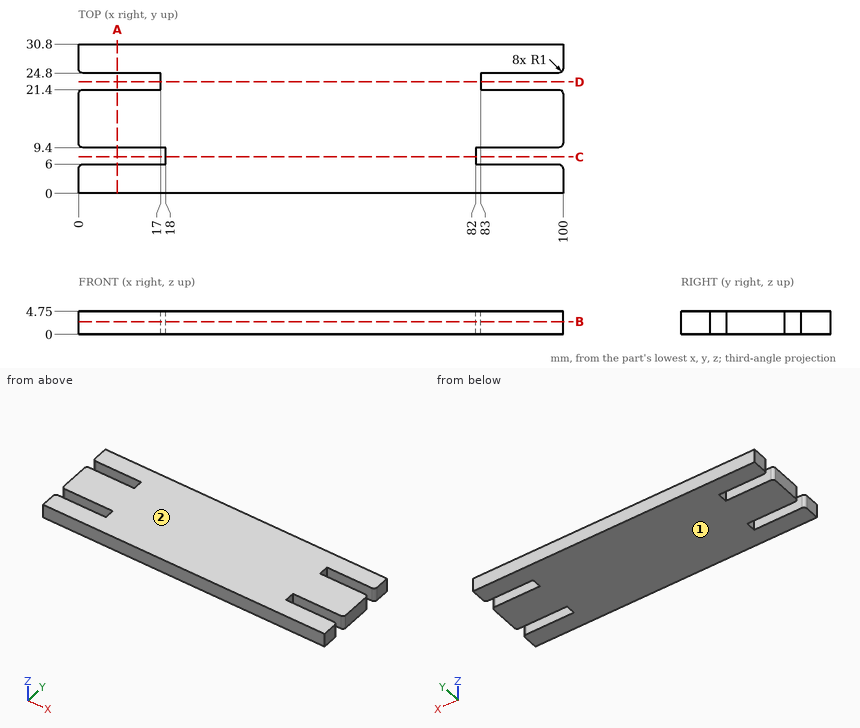
Verification items for this drawing (mm, ordinates from the low corner). Coordinates: 2 decimals unless noted, no trailing zeros. Write each loop counter-clockwise with the first axis right and the second up, starting at its lowest first coordinate (ties: lowest second). Pieces come first, ordered by that corner, then holes. Notation, with made-up numbers: (0.5, 88) -> (47.5, 88) arc R26 cw to (47.5, 119) -> close; hole circle Ø8 at (-8.75, 25.25). An arc over 180 degrees is marked (long way). One line per item, written item: value. Start each with the question number.
Q1. Thickness scan on L1, parallel to Y at x = 5, z = 3.8; L2, parallel to X at y = 9, z = 4.45; L3, parallel to X at y = 25, z = 3.95. Record the ranges inside material, lowest first. Write a range as from..to.
Q2. Go/stop test with flat-tipped pins: P1, Ø2.5, axis at y = 8, z = 3, coming from the -X side; P2, Ø2.5, axis at y = 7.5, z = 3.5, coming from the +X side; P3, Ø1, axis at y = 23, z = 3, coming from the -X side. Record where each tip stops, or that it passes through.
Q3. Cross-section at B-B on z = 2.6. Enter the section's corners in (x, y).
Q4. Cross-section at A-A on x = 8. Enter the section's corners in (y, z).
Q5. Cross-section at C-C on y = 7.5. Enter the section's corners in (x, z), and give its area (3 significant figures).
Q6. Cross-section at D-D on y = 23. Enter the section's corners in (x, z).
Q7. Mould release check, pull along Z, two halves, no side actions. Record for the marked faces 1 and 2: pulls with the +Z half, pulls with the -Z half, needs draft (parallel to the pull), parting line crosses it, or undercut.
Checked values:
1. L1: y = 0..6, 9.4..21.4, 24.8..30.8
1. L2: x = 18..82
1. L3: x = 0.4..99.6
2. P1: stops at x = 18
2. P2: stops at x = 82
2. P3: stops at x = 17
3. outline: (0, 0) -> (100, 0) -> (100, 5) arc R1 ccw to (99, 6) -> (82, 6) -> (82, 9.4) -> (99, 9.4) arc R1 ccw to (100, 10.4) -> (100, 20.4) arc R1 ccw to (99, 21.4) -> (83, 21.4) -> (83, 24.8) -> (99, 24.8) arc R1 ccw to (100, 25.8) -> (100, 30.8) -> (0, 30.8) -> (0, 25.8) arc R1 ccw to (1, 24.8) -> (17, 24.8) -> (17, 21.4) -> (1, 21.4) arc R1 ccw to (0, 20.4) -> (0, 10.4) arc R1 ccw to (1, 9.4) -> (18, 9.4) -> (18, 6) -> (1, 6) arc R1 ccw to (0, 5) -> close
4. outline: (0, 0) -> (6, 0) -> (6, 4.75) -> (0, 4.75) -> close; (9.4, 0) -> (21.4, 0) -> (21.4, 4.75) -> (9.4, 4.75) -> close; (24.8, 0) -> (30.8, 0) -> (30.8, 4.75) -> (24.8, 4.75) -> close
5. outline: (18, 0) -> (82, 0) -> (82, 4.75) -> (18, 4.75) -> close
5. area: 304 mm²
6. outline: (17, 0) -> (83, 0) -> (83, 4.75) -> (17, 4.75) -> close
7. face 1: pulls with the -Z half
7. face 2: pulls with the +Z half
